```python
from build123d import *

# Parameters (mm, degrees)
SKETCH_2_R               = 2.5
CUT_EXTRUDE_1_DEPTH      = 10
CUT_EXTRUDE_START        = -10
CUT_EXTRUDE_3_DEPTH      = 10
SKETCH_5_R               = 1.5
EXTRUDE_1_DEPTH          = 20.1
PATTERN_CIRCULAR_8_COUNT = 9


with BuildPart() as part:
    # ｽｹｯﾁ1 → 回転1 (revolve)
    with BuildSketch(Plane.XY, mode=Mode.PRIVATE) as revolve_1_sk:
        Polygon((-15, -3.484577548), (-15, -0.484577548), (-28.5, -0.484577548), (-28.5, 1.515422452), (-46, 1.515422452), (-46, -0.484577548), (-45.9999, -3.484577548), (-46, -5.484577548), (-28.5, -5.484577548), (-28.5, -3.484577548), align=None)
    revolve(revolve_1_sk.sketch.rotate(Axis((0, 0, 0), (0, 1, 0)), 270), axis=Axis((0, 0, 0), (0, 1, 0)))

    # ｽｹｯﾁ2 → ｶｯﾄ - 押し出し1 (cut)
    with BuildSketch(Plane(origin=(0, -0.484577548, 0), x_dir=(1, 0, 0), z_dir=(0, 1, 0))):
        with Locations(Location((0, 23.75, 0), (0, 0, 270))):
            Circle(SKETCH_2_R)
        with Locations(Location((20.56810334, 11.875, 0), (0, 0, 270))):
            Circle(SKETCH_2_R)
        with Locations(Location((20.56810334, -11.875, 0), (0, 0, 270))):
            Circle(SKETCH_2_R)
        with Locations(Location((0, -23.75, 0), (0, 0, 270))):
            Circle(SKETCH_2_R)
        with Locations(Location((-20.56810334, -11.875, 0), (0, 0, 270))):
            Circle(SKETCH_2_R)
        with Locations(Location((-20.56810334, 11.875, 0), (0, 0, 270))):
            Circle(SKETCH_2_R)
    extrude(amount=-CUT_EXTRUDE_1_DEPTH, mode=Mode.SUBTRACT)

    # ｽｹｯﾁ3 → ｶｯﾄ - 押し出し3 (cut)
    with BuildSketch(Plane(origin=(0, 1.515422452, 0), x_dir=(1, 0, 0), z_dir=(0, 1, 0)).offset(CUT_EXTRUDE_START)):
        with BuildLine():
            Line((4.340576232, 33.259012282), (2.102472879, 45.951927139))
            ThreePointArc((2.102472879, 45.951927139), (-7.987816173, 45.301156639), (-17.692162956, 42.461598768))
            Line((-17.692162956, 42.461598768), (-15.454059603, 29.768683911))
            ThreePointArc((-15.454059603, 29.768683911), (-14.63159697, 28.477676178), (-13.137147742, 28.14636476))
            Line((-13.137147742, 28.14636476), (2.718257082, 30.942100421))
            ThreePointArc((2.718257082, 30.942100421), (4.009264815, 31.764563054), (4.340576232, 33.259012282))
        make_face()
        with BuildLine():
            Line((8.0284955, 30.005762114), (21.9715045, 21.955762114))
            ThreePointArc((21.9715045, 21.955762114), (23.489142591, 21.755961269), (24.703555308, 22.687812921))
            Line((24.703555308, 22.687812921), (31.147917072, 33.849774919))
            ThreePointArc((31.147917072, 33.849774919), (23, 39.837168574), (13.740806456, 43.899774919))
            Line((13.740806456, 43.899774919), (7.296444692, 32.737812921))
            ThreePointArc((7.296444692, 32.737812921), (7.096643847, 31.220174831), (8.0284955, 30.005762114))
        make_face()
        with BuildLine():
            ThreePointArc((45.618904696, 5.908936816), (43.225860556, 15.732926593), (38.744299816, 24.796758494))
            Line((38.744299816, 24.796758494), (26.632861425, 20.388555425))
            ThreePointArc((26.632861425, 20.388555425), (25.504286137, 19.354406707), (25.43751647, 17.825129897))
            Line((25.43751647, 17.825129897), (30.944040777, 2.696078702))
            ThreePointArc((30.944040777, 2.696078702), (31.978189495, 1.567503415), (33.507466306, 1.500733748))
            Line((33.507466306, 1.500733748), (45.618904696, 5.908936816))
        make_face()
        with BuildLine():
            ThreePointArc((38.744299816, -24.796758494), (43.225860556, -15.732926593), (45.618904696, -5.908936816))
            Line((45.618904696, -5.908936816), (33.507466306, -1.500733748))
            ThreePointArc((33.507466306, -1.500733748), (31.978189495, -1.567503415), (30.944040777, -2.696078702))
            Line((30.944040777, -2.696078702), (25.43751647, -17.825129897))
            ThreePointArc((25.43751647, -17.825129897), (25.504286137, -19.354406707), (26.632861425, -20.388555425))
            Line((26.632861425, -20.388555425), (38.744299816, -24.796758494))
        make_face()
        with BuildLine():
            ThreePointArc((13.740806456, -43.899774919), (23, -39.837168574), (31.147917072, -33.849774919))
            Line((31.147917072, -33.849774919), (24.703555308, -22.687812921))
            ThreePointArc((24.703555308, -22.687812921), (23.489142591, -21.755961269), (21.9715045, -21.955762114))
            Line((21.9715045, -21.955762114), (8.0284955, -30.005762114))
            ThreePointArc((8.0284955, -30.005762114), (7.096643847, -31.220174831), (7.296444692, -32.737812921))
            Line((7.296444692, -32.737812921), (13.740806456, -43.899774919))
        make_face()
        with BuildLine():
            ThreePointArc((-17.692162956, -42.461598768), (-7.987816173, -45.301156639), (2.102472879, -45.951927139))
            Line((2.102472879, -45.951927139), (4.340576232, -33.259012282))
            ThreePointArc((4.340576232, -33.259012282), (4.009264815, -31.764563054), (2.718257082, -30.942100421))
            Line((2.718257082, -30.942100421), (-13.137147742, -28.14636476))
            ThreePointArc((-13.137147742, -28.14636476), (-14.63159697, -28.477676178), (-15.454059603, -29.768683911))
            Line((-15.454059603, -29.768683911), (-17.692162956, -42.461598768))
        make_face()
        with BuildLine():
            Line((-30.973437657, -12.870456857), (-40.846772695, -21.155168645))
            ThreePointArc((-40.846772695, -21.155168645), (-35.238044383, -29.568230046), (-27.92674174, -36.552661952))
            Line((-27.92674174, -36.552661952), (-18.053406702, -28.267950163))
            ThreePointArc((-18.053406702, -28.267950163), (-17.346592526, -26.910172763), (-17.806893036, -25.450286058))
            Line((-17.806893036, -25.450286058), (-28.155773552, -13.116970523))
            ThreePointArc((-28.155773552, -13.116970523), (-29.513550952, -12.410156347), (-30.973437657, -12.870456857))
        make_face()
        with BuildLine():
            Line((-32, 10.05), (-44.888723528, 10.05))
            ThreePointArc((-44.888723528, 10.05), (-46, 0), (-44.888723528, -10.05))
            Line((-44.888723528, -10.05), (-32, -10.05))
            ThreePointArc((-32, -10.05), (-30.585786438, -9.464213562), (-30, -8.05))
            Line((-30, -8.05), (-30, 8.05))
            ThreePointArc((-30, 8.05), (-30.585786438, 9.464213562), (-32, 10.05))
        make_face()
        with BuildLine():
            Line((-18.053406702, 28.267950163), (-27.92674174, 36.552661952))
            ThreePointArc((-27.92674174, 36.552661952), (-35.238044383, 29.568230046), (-40.846772695, 21.155168645))
            Line((-40.846772695, 21.155168645), (-30.973437657, 12.870456857))
            ThreePointArc((-30.973437657, 12.870456857), (-29.513550952, 12.410156347), (-28.155773552, 13.116970523))
            Line((-28.155773552, 13.116970523), (-17.806893036, 25.450286058))
            ThreePointArc((-17.806893036, 25.450286058), (-17.346592526, 26.910172763), (-18.053406702, 28.267950163))
        make_face()
    extrude(amount=CUT_EXTRUDE_3_DEPTH, mode=Mode.SUBTRACT)

    # ｽｹｯﾁ5 → ﾎﾞｽ - 押し出し1 (add)
    with BuildSketch(Plane(origin=(-9.897317918, 0, 1.745164186), x_dir=(-0.1736481776669516, 0, -0.9848077530122044), z_dir=(0.9848077530122044, 0, -0.1736481776669516))):
        with Locations((40.55, -1.984577548)):
            Circle(SKETCH_5_R)
    extrude_1 = extrude(amount=EXTRUDE_1_DEPTH)

    # 円形ﾊﾟﾀｰﾝ8: ﾎﾞｽ - 押し出し1 ×9 about axis
    pattern_circular_8_axis = Axis((0, 0, 0), (0, -1, 0))
    for i in range(1, PATTERN_CIRCULAR_8_COUNT):
        add(extrude_1.rotate(pattern_circular_8_axis, i * 360 / PATTERN_CIRCULAR_8_COUNT))


solid = part.part
```
Design review of the part built by this model. Coordinates are the model's own, in mm. A direction names the side the tool comes from. Round coordinates to 2 decimals unless told otherwise and drop trailing zeros. Write each loop counter-clockwise with the first axis right and the second up, starting at its lowest first coordinate (ties: lowest second). Pieces come first, ordered by that corner, then holes.
Item 1: For faces 4 (the cylindrical face through (-43.254, -1.02, 15.655)), 5 (the flat face through (14.9, -2.03, -26.04)), list the 3-axis set-ups (+Z, -Z, +X, -X, +Y, -Y) from which the entire face can be reached by the end or side of a thin tool; tool diameter is ignored.
Item 2: For probe 1 along Z at (x, y) = (38, 1.25); probe 2 along X at (y, z) = (-1.65, 0); probe 3 along Z at (x, y) = (-8, -1), list the stretches that pass through material, from the lowest coordinate up.
Item 3: We need section B-B on x = -11. State how many separate pieces and enclosed holes the cut face has, and give its area (3 significant figures).
Item 4: The part is to be moulded in two halves that separate along X. For faces 1 (the flat face through (15.098, -2.034, 25.924)), 2 (the cylindrical face through (-43.2, -1, -15.8)), 3 (the cylindrical face through (8.069, -4.499, -45.287)), say which applies: +X half, -X half, draft (parallel to the pull), parting line (faces both ways), or undercut.
Item 5: Clearance check with flat-ended pins moving along their axes: pin 1 Ø6.5 at (x, z) = (20.57, 11.88) entering from -Y; pin 2 Ø6.5 at (x, z) = (-20.57, 11.88) entering from +Y; pin 3 Ø1 at (x, y) = (15, -2.5) entering from -Z; pin 4 Ø4 at (x, z) = (0, -23.75) entering from -Y. State where each tip first meets the part, or that it passes through.
Item 6: We need section A-A on z = 0. Write out the cut boundary in (x, y), and give its area (3 significant figures).
Returned:
1. face 4: +Z, -X, +Y, -Y
1. face 5: +Y, -Y
2. probe 1: z = -25.92 to -24.53, -3.14 to 3.14, 24.53 to 25.92
2. probe 2: x = -42.01 to -39.09, -30 to -15, 15 to 46
2. probe 3: z = -40.91 to -38.62, -29.05 to -12.69, 12.69 to 29.05, 38.62 to 40.91
3. separate pieces: 4
3. enclosed holes: 0
3. area: 142 mm2
4. face 1: undercut
4. face 2: -X half
4. face 3: +X half
5. pin 1: stops at y = -3.48
5. pin 2: stops at y = -0.48
5. pin 3: stops at z = -40.12
5. pin 4: passes through
6. outline: circle Ø3 at (-40.55, -1.98); (-30, -5.48) - (-28.5, -5.48) - (-28.5, -3.48) - (-15, -3.48) - (-15, -0.48) - (-28.5, -0.48) - (-28.5, 1.52) - (-30, 1.52) - close; (15, -3.48) - (28.5, -3.48) - (28.5, -5.48) - (46, -5.48) - (46, 1.52) - (28.5, 1.52) - (28.5, -0.48) - (15, -0.48) - close
6. area: 221 mm2
